Study the drawing (mm; zero at the part's minimum x, y, z) and answer. A direction names the side the tool comes from. Coordinates: 2 decimals unless noted, no trailing zeros. Write each loop counter-clockwise with the first axis right and the second up, starting at its lowest first coordinate (ties: lowest second). Pieces come first, ordered by that corner, then holes. Notation, with made-up numbers: (83, -20) -> (103, -20) arc R11 cw to (103, -16) -> close; hole circle Ø5 at (-30, 65.25). An arc over 180 degrees is marked (long way). Write item = value, one per line. Start each with the question number.
1) Flat-ended cylindrical pins translate along their axes: pin 1 Ø3 at (y, z) = (296.5, 167) entering from -X; pin 2 Ø3 at (x, y) = (565.5, 195) entering from +Z; pin 3 Ø2 at (y, z) = (80.5, 147.5) entering from +X; pin 4 Ø3 at (x, y) = (219, 137.5) entering from -Z. Find the tip coordinate at first contact, or state that the pin passes through.
2) Section C-C (x = 378) is taken. Determine the outline of the cut face in (y, z), plus the area to 3 significant figures.
3) A tool of negligible diameter and unlimited length cuts with its end or side. For the marked faces 1 and 2, from which of +Z, -Z, +X, -X, +Y, -Y can it reach the whole face along a straight path? Write none if from no direction.
4) Section D-D (z = 29) is taken. Determine the outline of the cut face in (x, y), plus the area to 3 significant figures.
5) Section B-B (z = 100) is taken. Determine the outline of the cut face in (x, y), plus the area to 3 significant figures.
6) Find the intervals of material crossed by line 1 along X through (y, z) = (3, 100); line 2 along Z through (x, y) = (339, 257); line 3 along X through (y, z) = (6, 100), in increasing order. Write a range as from..to.
7) Section A-A (y = 300) is taken. Determine the outline of the cut face in (x, z).
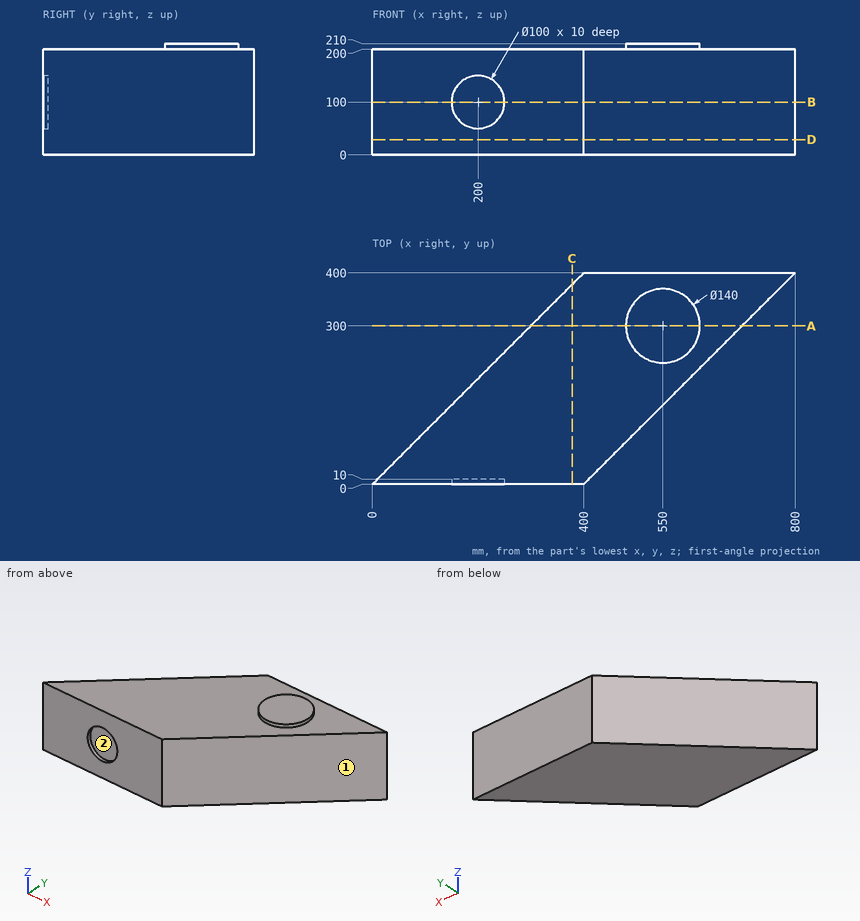
Answer key:
q1.pin_1 = 295
q1.pin_2 = 200
q1.pin_3 = 481.5
q1.pin_4 = 0
q2.outline = (0, 0) -> (378, 0) -> (378, 200) -> (0, 200) -> close
q2.area = 75,600 mm^2
q3.face_1 = +Z, -Z, +X, -Y
q3.face_2 = -Y
q4.outline = (0, 0) -> (400, 0) -> (800, 400) -> (400, 400) -> close
q4.area = 160,000 mm^2
q5.outline = (0, 0) -> (150, 0) -> (150, 10) -> (250, 10) -> (250, 0) -> (400, 0) -> (800, 400) -> (400, 400) -> close
q5.area = 159,000 mm^2
q6.line_1 = 3..150, 250..403
q6.line_2 = 0..200
q6.line_3 = 6..150, 250..406
q7.outline = (300, 0) -> (700, 0) -> (700, 200) -> (620, 200) -> (620, 210) -> (480, 210) -> (480, 200) -> (300, 200) -> close
